```python
from build123d import *

# Parameters (mm, degrees)
PAD_DEPTH    = 15
SKETCH001_W  = 10
SKETCH001_H  = 12
PAD001_DEPTH = 12.5
SKETCH002_R  = 0.625
POCKET_DEPTH = 5
SKETCH003_R  = 2
PAD002_DEPTH = 0.6
SKETCH004_R  = 1.5
PAD003_DEPTH = 9.4


with BuildPart() as part:
    # Sketch → Pad (new body)
    with BuildSketch(Plane.XY):
        with BuildLine():
            Line((-5, 3.5), (-5, -3.5))
            ThreePointArc((-5, -3.5), (0, -6), (5, -3.5))
            Line((5, 3.5), (5, -3.5))
            ThreePointArc((5, 3.5), (0, 6), (-5, 3.5))
        make_face()
    extrude(amount=PAD_DEPTH)

    # Sketch001 → Pad001 (new body)
    with BuildSketch(Plane.XY.offset(15)):
        Rectangle(SKETCH001_W, SKETCH001_H)
    extrude(amount=PAD001_DEPTH)

    # Sketch002 → Pocket (cut)
    with BuildSketch(Plane.XY.offset(27.5)):
        with Locations((0, -4.5)):
            Circle(SKETCH002_R)
        with Locations((0, 4.5)):
            Circle(SKETCH002_R)
    extrude(amount=-POCKET_DEPTH, mode=Mode.SUBTRACT)

    # Sketch003 → Pad002 (new body)
    with BuildSketch(Plane.XY.offset(27.5)):
        Circle(SKETCH003_R)
    extrude(amount=PAD002_DEPTH)

    # Sketch004 → Pad003 (new body)
    with BuildSketch(Plane.XY.offset(28.1)):
        Circle(SKETCH004_R)
    extrude(amount=PAD003_DEPTH)


solid = part.part
```
Can you work these out from the model? Positions are in its coordinate system, mm. A direction names the side the tool comes from. Coordinates: 2 decimals unless noted, no trailing zeros. Loops run counter-clockwise (first coordinate to the right, second up) from the corner with the lowest first, then second, coordinate; pieces in that order, holes last.
Item 1: Please list where these lines run through material, in increasing order: L1, parallel to Y at x = 0, z = 24 (3 decimals); L2, parallel to Z at x = -2.25, y = -3; L3, parallel to Y at x = -0.25, z = 9 (3 decimals).
Answers below:
L1: y = -6 to -5.125, -3.875 to 3.875, 5.125 to 6
L2: z = 0 to 27.5
L3: y = -5.995 to 5.995
Item 2: I'm going to push flat-ended pins straight in: pin 1 (1 mm diameter, centred on x = 0, y = -4, fed in from +Z); pin 2 (1 mm diameter, centred on x = 0, y = 4.5, fed in from +Z). Where does each tip first touch, or does it pass through?
Answers below:
pin 1: stops at z = 27.5
pin 2: stops at z = 22.5
Item 3: Suppose I cut it at C-C (z = 30.5). Please give me the cut outline in (x, y), then the cut area to 3 significant figures.
Answers below:
outline: circle Ø3 at (0, 0)
area: 7.07 mm2
Item 4: If we mould it in two halves opening along X, with no side actions, what happens to faces 6 (the face through (0, 4.5, 22.5)), 7 (the face through (0, 6, 7)), 8 (the face through (2.2, 0.1, 27.5)), 9 (the face through (0.596, -4.312, 25.035))? For each: released by +X, released by -X, zero draft, split by the parting line, or undercut.
Answers below:
face 6: undercut
face 7: split by the parting line
face 8: zero draft
face 9: undercut
Item 5: Suppose I cut it at D-D (y = -4.5). Please give me the cut outline in (x, z) (3 decimals), then the cut area to 3 significant figures.
Answers below:
outline: (-5, 15) - (-4.062, 15) - (-4.062, 0) - (4.062, 0) - (4.062, 15) - (5, 15) - (5, 27.5) - (0.625, 27.5) - (0.625, 22.5) - (-0.625, 22.5) - (-0.625, 27.5) - (-5, 27.5) - close
area: 241 mm2
Item 6: Suppose I cut it at B-B (x = -4). Please give me the cut outline in (y, z).
Answers below:
outline: (-6, 15) - (-4.55, 15) - (-4.55, 0) - (4.55, 0) - (4.55, 15) - (6, 15) - (6, 27.5) - (-6, 27.5) - close
Item 7: Which directions (+Z, -Z, +X, -X, +Y, -Y) give clear straight access to the entire face, cutting with the end or side of a thin tool? Please do faces 1 (the face through (-4, -5, 15)), 2 (the face through (4, 5, 15)), 3 (the face through (4, -5, 15)), 4 (the face through (-1.5, 0.07, 32.73)), 5 (the face through (0, -6, 7)).
Answers below:
face 1: -Z, -X, -Y
face 2: -Z, +X, +Y
face 3: -Z, +X, -Y
face 4: +Z
face 5: -Z, -Y
Item 8: Suppose I cut it at A-A (y = 0). Please give me the cut outline in (x, z).
Answers below:
outline: (-5, 0) - (5, 0) - (5, 27.5) - (2, 27.5) - (2, 28.1) - (1.5, 28.1) - (1.5, 37.5) - (-1.5, 37.5) - (-1.5, 28.1) - (-2, 28.1) - (-2, 27.5) - (-5, 27.5) - close
